CAD build for the part. Positions are in the model's coordinates, mm. Give positions to 0.01 mm unless a question says otherwise; leave off trailing zeros. Order: outer loops, then holes, each group sorted by start corner. A loop starts at its lowest first (then second) coordinate and runs counter-clockwise, first axis right, second up. Notation, with made-up numbers: (84.25, 58) -> (124.25, 58) arc R17 ccw to (124.25, 66) -> close; hole circle Ø11 at (13, 87.5). An arc over 180 degrees is marked (long way). Answer as CSV lines item,"result".
```python
from build123d import *

# Parameters (mm, degrees)
SKETCH1_W           = 87
SKETCH1_H           = 10
BOSS_EXTRUDE1_DEPTH = 10
SKETCH2_R           = 2.5
CUT_EXTRUDE1_DEPTH  = 4


with BuildPart() as part:
    # Sketch1 → Boss-Extrude1 (new body)
    with BuildSketch(Plane(origin=(0, 0, 0), x_dir=(1, 0, 0), z_dir=(0, 1, 0))):
        Rectangle(SKETCH1_W, SKETCH1_H)
    extrude(amount=BOSS_EXTRUDE1_DEPTH)

    # Sketch2 → Cut-Extrude1 (cut)
    with BuildSketch(Plane(origin=(43.5, 0, 0), x_dir=(0, 0, -1), z_dir=(1, 0, 0))):
        with Locations((0, 5)):
            Circle(SKETCH2_R)
    cut_extrude1 = extrude(amount=-CUT_EXTRUDE1_DEPTH, mode=Mode.SUBTRACT)

    # Mirror1: Cut-Extrude1 across plane
    add(cut_extrude1.mirror(Plane(origin=(0, 0, 0), x_dir=(0, 0, 1), z_dir=(1, 0, 0))), mode=Mode.SUBTRACT)


solid = part.part
```
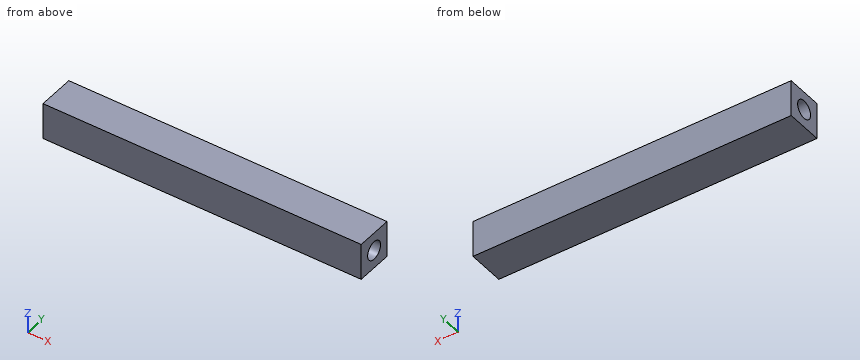
1) Wall check: line 1 along Y through (x, z) = (40.9, 0); line 2 along X through (y, z) = (5.5, -1.75). Give the ranges that are in metal, low to high. Write a range as [from, to].
Data:
line 1,"y = [0, 2.5], [7.5, 10]"
line 2,"x = [-39.5, 39.5]"
2) Band-saw the part on A-A, the plane z = -1.5. Write the cut outline in (x, y), then the cut area to 3 significant figures.
Data:
outline,"(-43.5, 0) -> (43.5, 0) -> (43.5, 3) -> (39.5, 3) -> (39.5, 7) -> (43.5, 7) -> (43.5, 10) -> (-43.5, 10) -> (-43.5, 7) -> (-39.5, 7) -> (-39.5, 3) -> (-43.5, 3) -> close"
area,"838 mm2"
3) Band-saw the part on B-B, the plane y = 5. Write the cut outline in (x, z), then the cut area to 3 significant figures.
Data:
outline,"(-43.5, -5) -> (43.5, -5) -> (43.5, -2.5) -> (39.5, -2.5) -> (39.5, 2.5) -> (43.5, 2.5) -> (43.5, 5) -> (-43.5, 5) -> (-43.5, 2.5) -> (-39.5, 2.5) -> (-39.5, -2.5) -> (-43.5, -2.5) -> close"
area,"830 mm2"
4) Pin check, flat tips, straight feed: P1, Ø3, axis at y = 5, z = 0, coming from the +X side; P2, Ø3, axis at y = 5, z = 0, coming from the -X side. Stop position of each tip, or through.
Data:
P1,"stops at x = 39.5"
P2,"stops at x = -39.5"
